The drawing under review shows one solid part. Ordinate dimensions are in mm from its lowest x, y, z. A direction names the side the tool comes from. Give positions to 0.01 mm unless a question says otherwise; leave off trailing zeros. Write each loop counter-clockwise with the first axis right and the second up, starting at its lowest first coordinate (ties: lowest second). Pieces come first, ordered by that corner, then holes. Notation, with made-up numbers: M 26.5,86 L 59.5,86 A26 ccw 59.5,109 Z; hole C -2,-32 d5. An arc over 180 degrees is marked long. Answer as a JSON object with one key per item and string values. Group by question number.
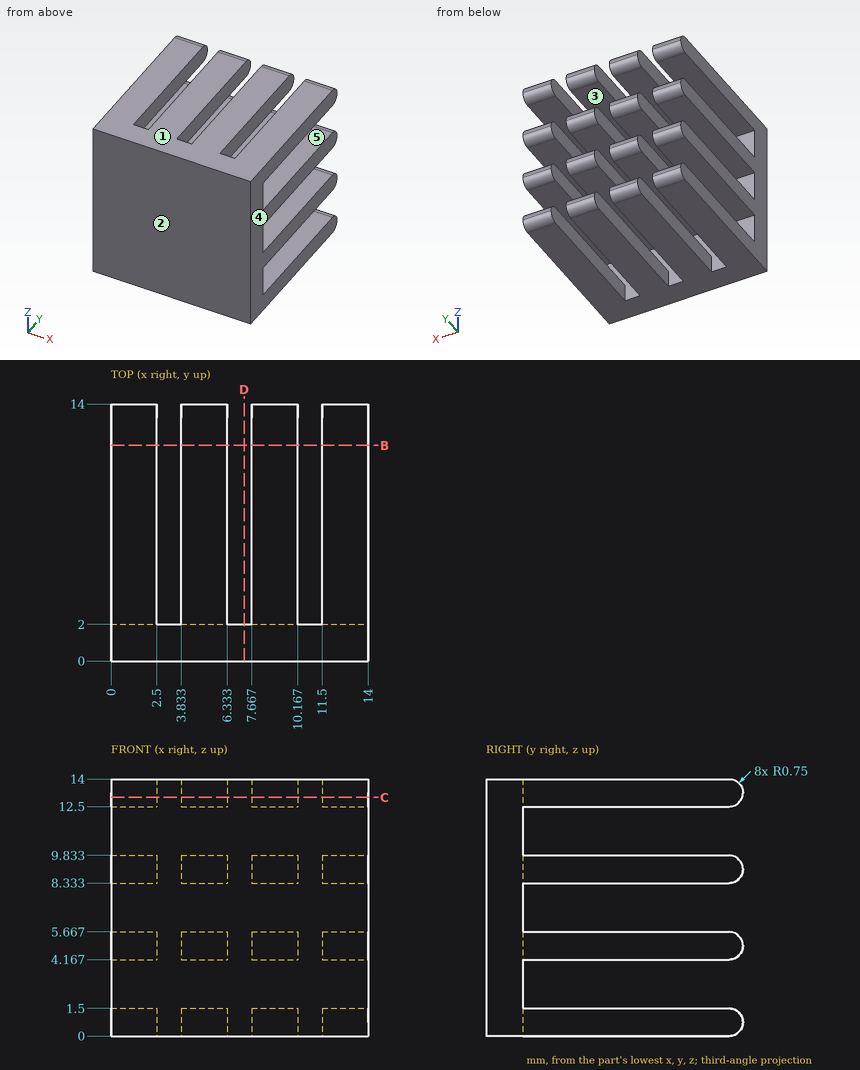
Item 1: Consider section C-C (z = 13). Give the boundary of the cut face in (x, y).
Item 2: Consider section D-D (x = 7.25). Give the boundary of the cut face in (y, z).
Item 3: Consider section B-B (y = 11.75). State how many separate pieces and enclosed holes the cut face has.
Item 4: Machinability: for the marked faces 4 and 5, which of the approach directions +Z, -Z, +X, -X, +Y, -Y give a long, thin tool a straight path to every point of the face, cutting with its end or side? Answer none if there is none.
Item 5: To check wall thickness, follow probe 1 along X at (y, z) = (6.25, 9.25); probe 2 along Z at (x, y) = (11.75, 11); probe 3 along Y at (x, z) = (9.5, 2.25). State the ranges of each line that lie inside material, in increasing order.
Item 6: Draft analysis for pull direction Z (two halves, no side actions). For the marked faces 1, 2 and 3, state which applies: released by +Z, released by -Z, zero draft, split by the parting line, or undercut.
Result set:
{
 "1": {"outline": "M 0,0 L 14,0 L 14,13.96 L 11.5,13.96 L 11.5,2 L 10.17,2 L 10.17,13.96 L 7.67,13.96 L 7.67,2 L 6.33,2 L 6.33,13.96 L 3.83,13.96 L 3.83,2 L 2.5,2 L 2.5,13.96 L 0,13.96 Z"},
 "2": {"outline": "M 0,0 L 2,0 L 2,14 L 0,14 Z"},
 "3": {"separate pieces": "16", "enclosed holes": "0"},
 "4": {"face 4": "+Z, -Z, +X, +Y, -Y", "face 5": "+X, -X, +Y"},
 "5": {"probe 1": "x = 0 to 2.5, 3.83 to 6.33, 7.67 to 10.17, 11.5 to 14", "probe 2": "z = 0 to 1.5, 4.17 to 5.67, 8.33 to 9.83, 12.5 to 14", "probe 3": "y = 0 to 2"},
 "6": {"face 1": "released by +Z", "face 2": "zero draft", "face 3": "undercut"}
}
